```python
from build123d import *

# Parameters (mm, degrees)
CROQUIS1_W                   = 43
CROQUIS1_H                   = 43
CROQUIS1_R                   = 13
CROQUIS1_R_2                 = 1.7
SALIENTE_EXTRUIR1_DEPTH      = 3.6
CROQUIS2_R                   = 2.95
CORTAR_EXTRUIR1_DEPTH        = 1.6
SALIENTE_EXTRUIR2_DEPTH      = 8
CROQUIS4_R                   = 1.7
CORTAR_EXTRUIR2_DEPTH        = 10
CORTAR_EXTRUIR3_DEPTH        = 1.5
CORTAR_EXTRUIR3_DEPTH_BACK   = 1.5
SALIENTE_EXTRUIR3_DEPTH      = 12.5
SALIENTE_EXTRUIR3_DEPTH_BACK = 12.5
CROQUIS8_R                   = 2.95
CORTAR_EXTRUIR4_DEPTH        = 3


with BuildPart() as part:
    # Croquis1 → Saliente-Extruir1 (new body)
    with BuildSketch(Plane.XY):
        Rectangle(CROQUIS1_W, CROQUIS1_H)
        Circle(CROQUIS1_R, mode=Mode.SUBTRACT)
        with Locations((-15.5, 15.5)):
            Circle(CROQUIS1_R_2, mode=Mode.SUBTRACT)
        with Locations((-15.5, -15.5)):
            Circle(CROQUIS1_R_2, mode=Mode.SUBTRACT)
        with Locations((15.5, -15.5)):
            Circle(CROQUIS1_R_2, mode=Mode.SUBTRACT)
        with Locations((15.5, 15.5)):
            Circle(CROQUIS1_R_2, mode=Mode.SUBTRACT)
    extrude(amount=SALIENTE_EXTRUIR1_DEPTH)

    # Croquis2 → Cortar-Extruir1 (cut)
    with BuildSketch(Plane.XY.offset(3.6)):
        with Locations((-15.5, 15.5)):
            Circle(CROQUIS2_R)
        with Locations((15.5, 15.5)):
            Circle(CROQUIS2_R)
        with Locations((-15.5, -15.5)):
            Circle(CROQUIS2_R)
        with Locations((15.5, -15.5)):
            Circle(CROQUIS2_R)
    extrude(amount=-CORTAR_EXTRUIR1_DEPTH, mode=Mode.SUBTRACT)

    # Croquis3 → Saliente-Extruir2 (add)
    with BuildSketch(Plane.XY.offset(3.6)):
        with BuildLine():
            Line((21.5, 2.6), (12.737346662, 2.6))
            ThreePointArc((12.737346662, 2.6), (12.241687471, 4.375052899), (11.5, 6.062177826))
            Line((11.5, 6.062177826), (11.5, 11))
            Line((11.5, 11), (21.5, 11))
            Line((21.5, 11), (21.5, 2.6))
        make_face()
    extrude(amount=SALIENTE_EXTRUIR2_DEPTH)

    # Croquis4 → Cortar-Extruir2 (cut)
    with BuildSketch(Plane.XZ.offset(-2.6)):
        with Locations((16.5, 7.6)):
            Circle(CROQUIS4_R)
    extrude(amount=-CORTAR_EXTRUIR2_DEPTH, mode=Mode.SUBTRACT)

    # Croquis6 → Cortar-Extruir3 (cut, two sides)
    with BuildSketch(Plane(origin=(0, 6.8, 0), x_dir=(-1, 0, 0), z_dir=(0, -1, 0))) as cortar_extruir3_sk:
        Polygon((-13.598814897, -9.275), (-13.598814897, -15.925), (-19.401185103, -15.925), (-19.401185103, -9.275), (-19.401185103, -5.925), (-16.5, -4.25), (-13.598814897, -5.925), align=None)
    extrude(amount=CORTAR_EXTRUIR3_DEPTH, mode=Mode.SUBTRACT)
    extrude(cortar_extruir3_sk.sketch, amount=-CORTAR_EXTRUIR3_DEPTH_BACK, mode=Mode.SUBTRACT)

    # Croquis7 → Saliente-Extruir3 (add, two sides)
    with BuildSketch(Plane(origin=(0, 0, 0), x_dir=(1, 0, 0), z_dir=(0, 1, 0))) as saliente_extruir3_sk:
        Polygon((-22.9, -7.7), (-18.5, -2.456284193), (-14.1, -7.7), align=None)
    extrude(amount=SALIENTE_EXTRUIR3_DEPTH)
    extrude(saliente_extruir3_sk.sketch, amount=-SALIENTE_EXTRUIR3_DEPTH_BACK)

    # Croquis8 → Cortar-Extruir4 (cut)
    with BuildSketch(Plane.XY.offset(3.6)):
        with Locations((-15.5, -15.5)):
            Circle(CROQUIS8_R)
        with Locations((-15.5, 15.5)):
            Circle(CROQUIS8_R)
    extrude(amount=-CORTAR_EXTRUIR4_DEPTH, mode=Mode.SUBTRACT)


solid = part.part
```
Check sheet for the modelled part. Datum: model origin and axes. Units: mm. A direction names the side the tool comes from. Give positions to 0.01 mm unless a question says otherwise; leave off trailing zeros. Write each loop counter-clockwise with the first axis right and the second up, starting at its lowest first coordinate (ties: lowest second). Pieces come first, ordered by that corner, then holes. Notation, with made-up numbers: (70.5, 17) - (128.5, 17) arc R22 cw to (128.5, 45) - close; hole circle Ø8 at (11, 5.25). An arc over 180 degrees is marked (long way). Answer as a JSON object with one key per item and string values. Group by question number.
1) Sectioned sample at C-C (x = -16.5). Record the cut outline in (y, z).
2) Sectioned sample at B-B (y = -15.5). Record the cut outline in (x, z), then the cut area to 3 significant figures.
3) Release check for a two-part mould opening along Y. For faces 1 (the face through (15, 11, 9)), 2 (the face through (-18.447, -15.37, 2.121)), 3 (the face through (9.3, -9.3, 0)) record: pulls with the +Y half, pulls with the -Y half, needs draft (parallel to the pull), parting line crosses it, or undercut.
4) Sectioned sample at D-D (x = 5). Record the cut outline in (y, z), then the cut area to 3 significant figures.
5) Thickness scan on probe 1 along X at (y, z) = (15.5, 0.45); probe 2 along Y at (x, z) = (-15.5, 1.4). Record the ranges inside material, lowest first. Write a range as from..to.
6) Depth check by flat-ended pin: P1, Ø1.8, axis at y = 3.5, z = 1.5, coming from the -X side; P2, Ø1.7, axis at x = 15.5, z = 8.5, coming from the +Y side; P3, Ø3, axis at y = 6.5, z = 6, coming from the -X side; P4, Ø3, axis at x = 15.5, y = -15.5, coming from the +Z side. Enter the tip coordinate at first touch or a pass-through.
7) Access from +Z, -Z, +X, -X, +Y, -Y to the whole of each face (thin tool, end or side, straight path). Record for faces 4 (the face through (-21.5, 0, 2)), 5 (the face through (16, 8.3, 10)), 6 (the face through (11.5, 8, 8)), 7 (the face through (17.07, -16.15, 0.99)).
8) Sectioned sample at A-A (x = 0). Record the cut outline in (y, z), then the cut area to 3 significant figures.
Geometry results:
{
 "1": {"outline": "(-21.5, 0) - (-16.87, 0) - (-16.87, 0.6) - (-18.28, 0.6) - (-18.28, 3.6) - (-21.5, 3.6) - close; (-14.13, 0) - (14.13, 0) - (14.13, 0.6) - (12.72, 0.6) - (12.72, 3.6) - (-12.72, 3.6) - (-12.72, 0.6) - (-14.13, 0.6) - close; (-12.5, 4.84) - (12.5, 4.84) - (12.5, 7.7) - (-12.5, 7.7) - close; (16.87, 0) - (21.5, 0) - (21.5, 3.6) - (18.28, 3.6) - (18.28, 0.6) - (16.87, 0.6) - close"},
 "2": {"outline": "(-21.5, 0) - (-17.2, 0) - (-17.2, 0.6) - (-18.45, 0.6) - (-18.45, 3.6) - (-21.5, 3.6) - close; (-13.8, 0) - (13.8, 0) - (13.8, 2) - (12.55, 2) - (12.55, 3.6) - (-12.55, 3.6) - (-12.55, 0.6) - (-13.8, 0.6) - close; (17.2, 0) - (21.5, 0) - (21.5, 3.6) - (18.45, 3.6) - (18.45, 2) - (17.2, 2) - close", "area": "119 mm^2"},
 "3": {"face 1": "pulls with the +Y half", "face 2": "undercut", "face 3": "needs draft"},
 "4": {"outline": "(-21.5, 0) - (-12, 0) - (-12, 3.6) - (-21.5, 3.6) - close; (12, 0) - (21.5, 0) - (21.5, 3.6) - (12, 3.6) - close", "area": "68.4 mm^2"},
 "5": {"probe 1": "x = -21.5..-17.2, -13.8..13.8, 17.2..21.5", "probe 2": "y = -21.5..-18.45, -12.55..12.55, 18.45..21.5"},
 "6": {"P1": "stops at x = -21.5", "P2": "stops at y = 11", "P3": "stops at x = -22.73", "P4": "passes through"},
 "7": {"face 4": "-Z, -X, +Y, -Y", "face 5": "+Z", "face 6": "+Z, +Y, -Y", "face 7": "+Z, -Z"},
 "8": {"outline": "(-21.5, 0) - (-13, 0) - (-13, 3.6) - (-21.5, 3.6) - close; (13, 0) - (21.5, 0) - (21.5, 3.6) - (13, 3.6) - close", "area": "61.2 mm^2"}
}
